Answer from the drawing. Dimensions are ordinates in mm from the lowest x, y and z of the part. Coordinates: 2 decimals unless noted, no trailing zeros. Order: outer loops, then holes, each group sorted by start corner. A loop starts at its lowest first (then second) coordinate and runs counter-clockwise, first axis right, second up. Notation, with made-up numbers: (74, 74.5) -> (85, 74.5) arc R8 ccw to (85, 84.5) -> close; hole circle Ø8 at (8, 54). An arc over 180 degrees is marked (long way). Answer in a Markdown table with one row per item.
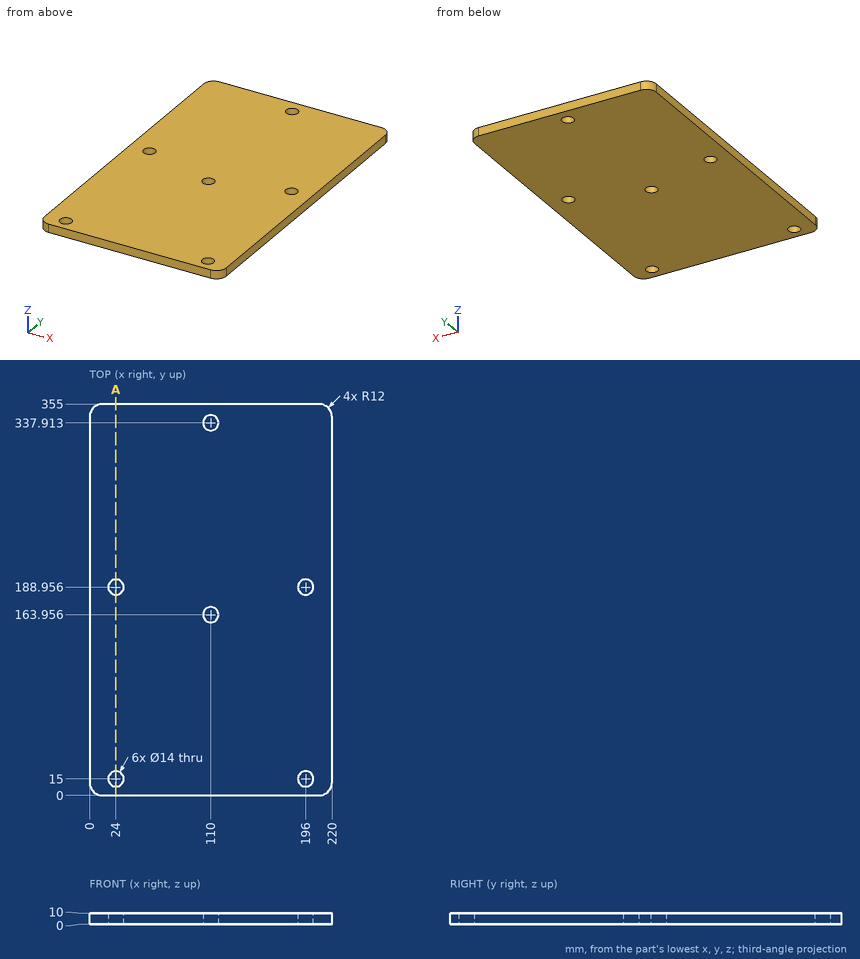
(1) Find the intervals of material crossed by line 1 along Y through (x, z) = (24, 5.25); line 2 along Y through (x, z) = (195.5, 3) (1 decimal); line 3 along X through (y, z) = (184.5, 1.5), in increasing order. Write a range as from..to.
Check values:
| item | result |
|---|---|
| line 1 | 0..8, 22..181.96, 195.96..355 |
| line 2 | 0..8, 22..182, 195.9..355 |
| line 3 | 0..18.6, 29.4..190.6, 201.4..220 |
(2) A flat-ended cylindrical pin translates along its axis: pin 1 (11 mm diameter, centred on x = 24, y = 15, fed in from +Z). Find the tip coordinate at first contact, or state that the pin passes through.
Check values:
| item | result |
|---|---|
| pin 1 | through |
(3) A cutting plane is placed at A-A, the plane x = 24. Determine the outline of the cut face in (y, z).
Check values:
| item | result |
|---|---|
| outline | (0, 0) -> (8, 0) -> (8, 10) -> (0, 10) -> close; (22, 0) -> (181.96, 0) -> (181.96, 10) -> (22, 10) -> close; (195.96, 0) -> (355, 0) -> (355, 10) -> (195.96, 10) -> close |
